Read the model definition and answer for the solid it produces. Units are mm, in the model's axes. A direction names the side the tool comes from. Coordinates: 2 decimals unless noted, no trailing zeros. Loops run counter-clockwise (first coordinate to the right, second up) from the corner with the lowest first, then second, coordinate; pieces in that order, holes last. Notation, with made-up numbers: M 7.5,39 L 66.5,39 A18 cw 66.5,50 Z; hole C 68,-34.5 d3. An arc over 180 degrees is marked long. One line per item, written item: value. Start each with the question number.
1. The part is cut by section A-A (x = 65.5). Write down the section's boundary in (y, z), then the cut area to 3 significant figures.
2. Determine the mould class of faces 1 (the face through (27, 51.03, -25)), 2 (the face through (23, 67, -44)), 3 (the face through (6, 59.084, -25)), 4 (the face through (68.75, 7.88, -2.01)) for opening direction Y: +Y half, -Y half, draft (parallel to the pull), parting line (faces both ways), or undercut.
3. The part is cut by section C-C (y = 55). Write down the section's boundary in (x, z), then the cut area to 3 significant figures.
4. Consider probe 1 along X at (y, z) = (8, -23); probe 2 along X at (y, z) = (34, -41); probe 3 along Y at (x, z) = (43, -5.5). Determine where each line is inside the solid, lowest interval first.
5. Flat-ended cylindrical pins translate along their axes: pin 1 (5 mm diameter, centred on x = 22, z = -10.5, fed in from -Y); pin 2 (8 mm diameter, centred on y = 64, z = -18, fed in from +X); pin 3 (4 mm diameter, centred on y = 40.5, z = -40.5, fed in from +X). Find the tip coordinate at first contact, or state that the pin passes through.
6. For faces 5 (the face through (18, 13, -48)), 6 (the face through (61.924, 6, -25)), 7 (the face through (23, 6, -4.084)), 8 (the face through (41, 71.03, -25)), 9 (the face through (6, 12.424, -25)), determine the directions among +Z, -Z, +X, -X, +Y, -Y from which every point of the face is accessible in a straight line to the end or side of a thin tool.
7. The part is cut by section B-B (z = -15). State how many separate pieces and enclosed holes the cut face has, then the cut area to 3 significant figures.
```python
from build123d import *

# Parameters (mm, degrees)
SKETCH1_W           = 109
SKETCH1_H           = 50
BOSS_EXTRUDE1_DEPTH = 13
SKETCH2_W           = 20.172406269
SKETCH2_H           = 41.768023424
SKETCH2_W_2         = 20.8632421
SKETCH2_W_3         = 7.295226376
SKETCH2_W_4         = 7.129425777
CUT_EXTRUDE1_DEPTH  = 16
SKETCH4_W           = 12.874624242
SKETCH4_H           = 50
SKETCH4_W_2         = 10.390561779
BOSS_EXTRUDE2_DEPTH = 47.03
SKETCH5_W           = 50
SKETCH5_H           = 13
BOSS_EXTRUDE3_DEPTH = 46
SKETCH6_W           = 8.994074375
SKETCH6_H           = 50
CUT_EXTRUDE2_DEPTH  = 2
SKETCH7_W           = 17.404486576
SKETCH7_H           = 39
CUT_EXTRUDE3_DEPTH  = 22
SKETCH8_W           = 30.430427264
SKETCH8_H           = 46.659988472
CUT_EXTRUDE4_DEPTH  = 22
SKETCH9_R           = 1.9
CUT_EXTRUDE5_DEPTH  = 60


with BuildPart() as part:
    # Sketch1 → Boss-Extrude1 (new body)
    with BuildSketch(Plane(origin=(0, 0, 0), x_dir=(1, 0, 0), z_dir=(0, 1, 0))):
        with Locations((54.5, 25)):
            Rectangle(SKETCH1_W, SKETCH1_H)
    extrude(amount=BOSS_EXTRUDE1_DEPTH)

    # Sketch2 → Cut-Extrude1 (cut)
    with BuildSketch(Plane(origin=(0, 0, 0), x_dir=(-1, 0, 0), z_dir=(0, -1, 0))):
        with Locations((-22.960827377, 24.968248552)):
            Rectangle(SKETCH2_W, SKETCH2_H)
        with Locations((-72.355589302, 24.968248552)):
            Rectangle(SKETCH2_W_2, SKETCH2_H)
        with Locations((-47.402599082, 24.968248552)):
            Rectangle(SKETCH2_W_3, SKETCH2_H)
        with Locations((-96.396676226, 24.968248552)):
            Rectangle(SKETCH2_W_4, SKETCH2_H)
    extrude(amount=-CUT_EXTRUDE1_DEPTH, mode=Mode.SUBTRACT)

    # Sketch4 → Boss-Extrude2 (add)
    with BuildSketch(Plane(origin=(0, 13, 0), x_dir=(1, 0, 0), z_dir=(0, 1, 0))):
        with Locations((6.437312121, 25)):
            Rectangle(SKETCH4_W, SKETCH4_H)
        with Locations((29.461633581, 25)):
            Rectangle(SKETCH4_W_2, SKETCH4_H)
    extrude(amount=BOSS_EXTRUDE2_DEPTH)

    # Sketch5 → Boss-Extrude3 (add)
    with BuildSketch(Plane.ZY):
        with Locations((-25, 66.53)):
            Rectangle(SKETCH5_W, SKETCH5_H)
    extrude(amount=-BOSS_EXTRUDE3_DEPTH)

    # Sketch6 → Cut-Extrude2 (cut)
    with BuildSketch(Plane(origin=(0, 73.03, 0), x_dir=(1, 0, 0), z_dir=(0, 1, 0))):
        with Locations((41.502962813, 25)):
            Rectangle(SKETCH6_W, SKETCH6_H)
    extrude(amount=-CUT_EXTRUDE2_DEPTH, mode=Mode.SUBTRACT)

    # Sketch7 → Cut-Extrude3 (cut)
    with BuildSketch(Plane(origin=(0, 73.03, 0), x_dir=(1, 0, 0), z_dir=(0, 1, 0))):
        with Locations((20.762468631, 24.5)):
            Rectangle(SKETCH7_W, SKETCH7_H)
    extrude(amount=-CUT_EXTRUDE3_DEPTH, mode=Mode.SUBTRACT)

    # Sketch8 → Cut-Extrude4 (cut)
    with BuildSketch(Plane.ZY):
        with Locations((-24.949282621, 35.754239318)):
            Rectangle(SKETCH8_W, SKETCH8_H)
    extrude(amount=-CUT_EXTRUDE4_DEPTH, mode=Mode.SUBTRACT)

    # Sketch9 → Cut-Extrude5 (cut)
    with BuildSketch(Plane.XY):
        with Locations((21.57993313, 65.011863681)):
            Circle(SKETCH9_R)
        with Locations((21.57863067, 8.007764563)):
            Circle(SKETCH9_R)
        with Locations((70.65, 7.798014497)):
            Circle(SKETCH9_R)
    extrude(amount=-CUT_EXTRUDE5_DEPTH, mode=Mode.SUBTRACT)


solid = part.part
```
Answer block:
1. outline: M 0,-50 L 13,-50 L 13,-45.85 L 0,-45.85 Z; M 0,-4.08 L 13,-4.08 L 13,0 L 0,0 Z
1. area: 107 mm2
2. face 1: +Y half
2. face 2: draft
2. face 3: undercut
2. face 4: undercut
3. outline: M 0,-50 L 12.87,-50 L 12.87,-44 L 12.06,-44 L 12.06,-40.16 L 0,-40.16 Z; M 0,-9.73 L 12.06,-9.73 L 12.06,-5 L 12.87,-5 L 12.87,0 L 0,0 Z; M 24.27,-50 L 34.66,-50 L 34.66,0 L 24.27,0 L 24.27,-5 L 29.46,-5 L 29.46,-44 L 24.27,-44 Z
3. area: 562 mm2
4. probe 1: x = 0 to 12.87, 33.05 to 43.75, 51.05 to 61.92, 82.79 to 92.83, 99.96 to 109
4. probe 2: x = 0 to 12.87, 24.27 to 34.66
4. probe 3: y = 0 to 13, 60.03 to 71.03
5. pin 1: stops at y = 13
5. pin 2: stops at x = 46
5. pin 3: stops at x = 34.66
6. face 5: +Z, -Z
6. face 6: +Y, -Y
6. face 7: -Y
6. face 8: +Z, -Z, +X, +Y
6. face 9: -X
7. separate pieces: 6
7. enclosed holes: 0
7. area: 1,500 mm2
